Can you work these out from the model? Positions are in its coordinate system, mm. A direction names the side the tool comes from. Round coordinates to 2 decimals unless told otherwise and drop trailing zeros. Loops run counter-clockwise (first coordinate to the right, second up) from the corner with the lowest first, then second, coordinate; pieces in that order, holes last. Notation, with made-up numbers: M 38.25,11.5 L 69.25,11.5 A32 cw 69.25,39.5 Z; hole C 54.5,48 d2. An arc over 180 degrees is marked long. Return JSON: item names as keys, results as strings.
```python
from build123d import *

# Parameters (mm, degrees)
SKETCH_W                         = 14
SKETCH_H                         = 42
PAD_DEPTH                        = 14
SKETCH001_W                      = 13
SKETCH001_H                      = 40
POCKET_DEPTH                     = 8
SKETCH002_W                      = 8.5
SKETCH002_H                      = 24.5
POCKET001_DEPTH                  = 5
SKETCH003_W                      = 6
SKETCH003_H                      = 7
POCKET002_DEPTH                  = 5
SKETCH004_R                      = 1
POCKET003_DEPTH                  = 5
SKETCH004_LINEARPATTERN_2_R      = 1
POCKET003_LINEARPATTERN_2_DEPTH  = 5
SKETCH004_LINEARPATTERN_3_R      = 1
POCKET003_LINEARPATTERN_3_DEPTH  = 5
SKETCH004_LINEARPATTERN_4_R      = 1
POCKET003_LINEARPATTERN_4_DEPTH  = 5
SKETCH004_LINEARPATTERN_5_R      = 1
POCKET003_LINEARPATTERN_5_DEPTH  = 5
SKETCH004_LINEARPATTERN_6_R      = 1
POCKET003_LINEARPATTERN_6_DEPTH  = 5
SKETCH004_LINEARPATTERN_7_R      = 1
POCKET003_LINEARPATTERN_7_DEPTH  = 5
SKETCH004_LINEARPATTERN_8_R      = 1
POCKET003_LINEARPATTERN_8_DEPTH  = 5
SKETCH004_LINEARPATTERN_9_R      = 1
POCKET003_LINEARPATTERN_9_DEPTH  = 5
SKETCH004_LINEARPATTERN_10_R     = 1
POCKET003_LINEARPATTERN_10_DEPTH = 5
LINEARPATTERN001_COUNT           = 3
LINEARPATTERN001_PITCH           = 2.5
SKETCH007_W                      = 4
SKETCH007_H                      = 2
PAD001_DEPTH                     = 3
SKETCH016_W                      = 3
SKETCH016_H                      = 40
POCKET007_DEPTH                  = 5


with BuildPart() as obj1:
    # Sketch → Pad (new body)
    with BuildSketch(Plane.XY):
        with Locations((7, 21)):
            Rectangle(SKETCH_W, SKETCH_H)
    extrude(amount=PAD_DEPTH)

    # Sketch001 (on Face6 of Pad) → Pocket (cut)
    with BuildSketch(Plane.XY.offset(14)):
        with Locations((6.5, 21)):
            Rectangle(SKETCH001_W, SKETCH001_H)
    extrude(amount=-POCKET_DEPTH, mode=Mode.SUBTRACT)

    # Sketch002 (on Face7 of Pocket) → Pocket001 (cut)
    with BuildSketch(Plane.XY.offset(6)):
        with Locations((4.25, 19.75)):
            Rectangle(SKETCH002_W, SKETCH002_H)
    extrude(amount=-POCKET001_DEPTH, mode=Mode.SUBTRACT)

    # Sketch003 (on Face6 of Pocket001) → Pocket002 (cut)
    with BuildSketch(Plane.XZ.offset(-41)):
        with Locations((3, 9.5)):
            Rectangle(SKETCH003_W, SKETCH003_H)
    extrude(amount=-POCKET002_DEPTH, mode=Mode.SUBTRACT)

    # Sketch004 (on Face16 of Pocket002) → Pocket003 (cut)
    with BuildSketch(Plane.XY.offset(1)):
        with Locations((6.5, 9.5)):
            Circle(SKETCH004_R)
    pocket003 = extrude(amount=-POCKET003_DEPTH, mode=Mode.SUBTRACT)

    # Sketch004 LinearPattern 2 → Pocket003 LinearPattern 2 (cut)
    with BuildSketch(Plane(origin=(0, 2.222222, 1), x_dir=(1, 0, 0), z_dir=(0, 0, 1))):
        with Locations((6.5, 9.5)):
            Circle(SKETCH004_LINEARPATTERN_2_R)
    pocket003_linearpattern_2 = extrude(amount=-POCKET003_LINEARPATTERN_2_DEPTH, mode=Mode.SUBTRACT)

    # Sketch004 LinearPattern 3 → Pocket003 LinearPattern 3 (cut)
    with BuildSketch(Plane(origin=(0, 4.444444, 1), x_dir=(1, 0, 0), z_dir=(0, 0, 1))):
        with Locations((6.5, 9.5)):
            Circle(SKETCH004_LINEARPATTERN_3_R)
    pocket003_linearpattern_3 = extrude(amount=-POCKET003_LINEARPATTERN_3_DEPTH, mode=Mode.SUBTRACT)

    # Sketch004 LinearPattern 4 → Pocket003 LinearPattern 4 (cut)
    with BuildSketch(Plane(origin=(0, 6.666667, 1), x_dir=(1, 0, 0), z_dir=(0, 0, 1))):
        with Locations((6.5, 9.5)):
            Circle(SKETCH004_LINEARPATTERN_4_R)
    pocket003_linearpattern_4 = extrude(amount=-POCKET003_LINEARPATTERN_4_DEPTH, mode=Mode.SUBTRACT)

    # Sketch004 LinearPattern 5 → Pocket003 LinearPattern 5 (cut)
    with BuildSketch(Plane(origin=(0, 8.888889, 1), x_dir=(1, 0, 0), z_dir=(0, 0, 1))):
        with Locations((6.5, 9.5)):
            Circle(SKETCH004_LINEARPATTERN_5_R)
    pocket003_linearpattern_5 = extrude(amount=-POCKET003_LINEARPATTERN_5_DEPTH, mode=Mode.SUBTRACT)

    # Sketch004 LinearPattern 6 → Pocket003 LinearPattern 6 (cut)
    with BuildSketch(Plane(origin=(0, 11.111111, 1), x_dir=(1, 0, 0), z_dir=(0, 0, 1))):
        with Locations((6.5, 9.5)):
            Circle(SKETCH004_LINEARPATTERN_6_R)
    pocket003_linearpattern_6 = extrude(amount=-POCKET003_LINEARPATTERN_6_DEPTH, mode=Mode.SUBTRACT)

    # Sketch004 LinearPattern 7 → Pocket003 LinearPattern 7 (cut)
    with BuildSketch(Plane(origin=(0, 13.333333, 1), x_dir=(1, 0, 0), z_dir=(0, 0, 1))):
        with Locations((6.5, 9.5)):
            Circle(SKETCH004_LINEARPATTERN_7_R)
    pocket003_linearpattern_7 = extrude(amount=-POCKET003_LINEARPATTERN_7_DEPTH, mode=Mode.SUBTRACT)

    # Sketch004 LinearPattern 8 → Pocket003 LinearPattern 8 (cut)
    with BuildSketch(Plane(origin=(0, 15.555556, 1), x_dir=(1, 0, 0), z_dir=(0, 0, 1))):
        with Locations((6.5, 9.5)):
            Circle(SKETCH004_LINEARPATTERN_8_R)
    pocket003_linearpattern_8 = extrude(amount=-POCKET003_LINEARPATTERN_8_DEPTH, mode=Mode.SUBTRACT)

    # Sketch004 LinearPattern 9 → Pocket003 LinearPattern 9 (cut)
    with BuildSketch(Plane(origin=(0, 17.777778, 1), x_dir=(1, 0, 0), z_dir=(0, 0, 1))):
        with Locations((6.5, 9.5)):
            Circle(SKETCH004_LINEARPATTERN_9_R)
    pocket003_linearpattern_9 = extrude(amount=-POCKET003_LINEARPATTERN_9_DEPTH, mode=Mode.SUBTRACT)

    # Sketch004 LinearPattern 10 → Pocket003 LinearPattern 10 (cut)
    with BuildSketch(Plane(origin=(0, 20, 1), x_dir=(1, 0, 0), z_dir=(0, 0, 1))):
        with Locations((6.5, 9.5)):
            Circle(SKETCH004_LINEARPATTERN_10_R)
    pocket003_linearpattern_10 = extrude(amount=-POCKET003_LINEARPATTERN_10_DEPTH, mode=Mode.SUBTRACT)

    # LinearPattern001: Pocket003, Pocket003 LinearPattern 2, Pocket003 LinearPattern 3, Pocket003 LinearPattern 4, Pocket003 LinearPattern 5, Pocket003 LinearPattern 6, Pocket003 LinearPattern 7, Pocket003 LinearPattern 8, Pocket003 LinearPattern 9, Pocket003 LinearPattern 10 ×3
    with Locations(*[(-i * LINEARPATTERN001_PITCH, 0, 0) for i in range(1, LINEARPATTERN001_COUNT)]):
        add(pocket003, mode=Mode.SUBTRACT)
        add(pocket003_linearpattern_2, mode=Mode.SUBTRACT)
        add(pocket003_linearpattern_3, mode=Mode.SUBTRACT)
        add(pocket003_linearpattern_4, mode=Mode.SUBTRACT)
        add(pocket003_linearpattern_5, mode=Mode.SUBTRACT)
        add(pocket003_linearpattern_6, mode=Mode.SUBTRACT)
        add(pocket003_linearpattern_7, mode=Mode.SUBTRACT)
        add(pocket003_linearpattern_8, mode=Mode.SUBTRACT)
        add(pocket003_linearpattern_9, mode=Mode.SUBTRACT)
        add(pocket003_linearpattern_10, mode=Mode.SUBTRACT)

    # Sketch007 → Pad001 (join)
    with BuildSketch(Plane(origin=(0, 1, 0), x_dir=(-1, 0, 0), z_dir=(0, 1, 0))):
        with Locations((-2, 8)):
            Rectangle(SKETCH007_W, SKETCH007_H)
    extrude(amount=PAD001_DEPTH)

    # Sketch016 (on Face44 of Pad001) → Pocket007 (cut)
    with BuildSketch(Plane.XY.offset(6)):
        with Locations((11.5, 21)):
            Rectangle(SKETCH016_W, SKETCH016_H)
    extrude(amount=-POCKET007_DEPTH, mode=Mode.SUBTRACT)


with BuildPart() as obj2:
    # Part__Mirroring: instance of obj1
    add(obj1.part.mirror(Plane(origin=(0, 0, 0), x_dir=(0, -1, 0), z_dir=(1, 0, 0))))


solid = obj2.part
```
Q1. Thinking about a two-plate mould opening in X: for faces 4 (the flat face through (-2, 4, 8)), 5 (the flat face through (0, 41.5, 13.5)), 6 (the cylindrical face through (-6.28, 24.08, 0.51)), which applies, pulls with the +X half, pulls with the -X half, needs draft (parallel to the pull), parting line crosses it, or undercut?
Results:
{"face 4": "needs draft", "face 5": "pulls with the +X half", "face 6": "undercut"}
Q2. Suppose I cut it at C-C, the plane z = 5.5. Please give me the cut outline in (x, y), plus the area to 3 significant figures.
Results:
{"outline": "M -14,0 L 0,0 L 0,7.5 L -8.5,7.5 L -8.5,32 L 0,32 L 0,42 L -14,42 Z; hole M -13,1 L -10,1 L -10,41 L -13,41 Z", "area": "260 mm2"}
Q3. Suppose I cut it at B-B, the plane x = -12.5. Please give me the cut outline in (y, z).
Results:
{"outline": "M 0,0 L 42,0 L 42,14 L 41,14 L 41,1 L 1,1 L 1,14 L 0,14 Z"}
Q4. I'm going to push flat-ended pins straight in: pin 1 Ø6 at (x, y) = (-4.5, 37) entering from +Z; pin 2 Ø1.5 at (x, y) = (-11.5, 17.5) entering from +Z; pin 3 Ø6 at (y, z) = (15, 8) entering from +X. Where does each tip first touch, or does it pass through?
Results:
{"pin 1": "stops at z = 6", "pin 2": "stops at z = 1", "pin 3": "stops at x = -8.5"}
Q5. Suppose I cut it at A-A, the plane y = 29.5. Please give me the cut outline in (x, z).
Results:
{"outline": "M -14,0 L -7.5,0 L -7.5,1 L -8.5,1 L -8.5,6 L -10,6 L -10,1 L -13,1 L -13,14 L -14,14 Z; M -5.5,0 L -5,0 L -5,1 L -5.5,1 Z; M -3,0 L -2.5,0 L -2.5,1 L -3,1 Z; M -0.5,0 L 0,0 L 0,1 L -0.5,1 Z"}
Q6. If I drill on line 1 along Y through (x, z) = (-2, 5.75); line 2 along X through (y, z) = (10, 1.25); line 3 along Y through (x, z) = (-11, 11), over which ranges is the centre line in solid material (lowest first)?
Results:
{"line 1": "y = 0 to 7.5, 32 to 42", "line 2": "x = -14 to -13, -10 to -8.5", "line 3": "y = 0 to 1, 41 to 42"}
Q7. On a 3-axis mill with a long thin cutter (end or side, diameter ignored), from which of +Z, -Z, +X, -X, +Y, -Y can I reach the whole of each face in a straight line? I mean faces 1 (the flat face through (-4, 7.5, 4)), 2 (the flat face through (-4, 2, 8)), 3 (the flat face through (-2, 2, 9)). Say none if no direction works.
Results:
{"face 1": "+Z, +X", "face 2": "+Z, +Y", "face 3": "+Z, +X, +Y"}
Q8. Suppose I cut it at D-D, the plane z = 10. Please give me the cut outline in (x, y).
Results:
{"outline": "M -14,0 L 0,0 L 0,1 L -13,1 L -13,41 L -6,41 L -6,42 L -14,42 Z"}
